Verification items for the finished model (mm, model axes). A direction names the side the tool comes from. Round coordinates to 2 decimals unless told otherwise and drop trailing zeros. Write each loop counter-clockwise with the first axis right and the second up, starting at its lowest first coordinate (ties: lowest second). Pieces come first, ordered by that corner, then holes.
from build123d import *

# Parameters (mm, degrees)
F0_W     = 9.545457
F0_H     = 70.051323
F1_DEPTH = 10
F3_DEPTH = 50
F0_W_2   = 6.466273
F4_DEPTH = 20
F6_DEPTH = 50


with BuildPart() as f1:
    # F0 (on Top) → F1 (new body)
    with BuildSketch(Plane.XY):
        with Locations((-40.414223, 12.239737)):
            Rectangle(F0_W, F0_H)
    extrude(amount=F1_DEPTH)

    # F2 (on Right) → F3 (cut)
    with BuildSketch(Plane.YZ):
        with BuildLine():
            ThreePointArc((-10.673997, 12.938293), (14.378322, 4.831678), (39.214806, 13.577245))
            Line((39.214806, 13.577245), (-10.673997, 12.938293))
        make_face()
    extrude(amount=-F3_DEPTH, mode=Mode.SUBTRACT)

    # F0 (on Top) → F4 (join)
    with BuildSketch(Plane.XY):
        with Locations((-32.408358, 12.239737)):
            Rectangle(F0_W_2, F0_H)
    extrude(amount=F4_DEPTH)

    # F5 (on Right) → F6 (cut)
    with BuildSketch(Plane.YZ):
        with BuildLine():
            Line((46.000224, 26.69229), (-19.578034, 26.722144))
            ThreePointArc((-19.578034, 26.722144), (13.203243, 9.459906), (46.000224, 26.69229))
        make_face()
    extrude(amount=-F6_DEPTH, mode=Mode.SUBTRACT)


solid = f1.part
Q1. Material ranges on line 1 along X through (y, z) = (33, 13.75); line 2 along Y through (x, z) = (-33.5, 18.5); line 3 along Z through (x, y) = (-40.25, 13), recorded low to high.
Recorded:
line 1: x = -35.64 to -29.18
line 2: y = -22.79 to -12.03, 38.47 to 47.27
line 3: z = 0 to 4.84
Q2. Sectioned sample at A-A (z = 13). Enter the section's corners in (x, y).
Recorded:
outline: (-35.64, -22.79) - (-29.18, -22.79) - (-29.18, -3.19) - (-35.64, -3.19) - close; (-35.64, 29.63) - (-29.18, 29.63) - (-29.18, 47.27) - (-35.64, 47.27) - close
Q3. Depth check by flat-ended pin: P1, Ø5, axis at y = 14.5, z = 10, coming from the +X side; P2, Ø3, axis at x = -35.5, y = 9.5, coming from the +Z side; P3, Ø6, axis at x = -40, y = 39.5, coming from the +Z side; P4, Ø5, axis at x = -43, z = 14, coming from the -Y side. Enter the tip coordinate at first touch or a pass-through.
Recorded:
P1: stops at x = -29.18
P2: stops at z = 9.8
P3: stops at z = 10
P4: passes through
Q4. Release check for a two-part mould opening along Y. For faces 4 (the flat face through (-40, -14, 10)), 5 (the flat face through (-36, 47.265, 8)), 6 (the flat face through (-35.641, 12, 9)) record: released by +Y, released by -Y, zero draft, split by the parting line, or undercut.
Recorded:
face 4: zero draft
face 5: released by +Y
face 6: undercut
Q5. Sectioned sample at B-B (x = -37.5). Enter the section's corners in (y, z).
Recorded:
outline: (-22.79, 0) - (47.27, 0) - (47.27, 10) - (33.82, 10) arc R41.14 cw to (-6.12, 10) - (-22.79, 10) - close
Q6. Tool access check on faces 1 (the flat face through (-32, 44, 20)), 2 (the flat face through (-40, 41, 10)), 3 (the cylindrical face through (-40.35, 13.56, 4.83)). Record the directions out of +Z, -Z, +X, -X, +Y, -Y that give a thin tool (end or side, any length) a straight path to the whole face; none if there is none.
Recorded:
face 1: +Z, +X, -X, +Y, -Y
face 2: +Z, -X, +Y, -Y
face 3: +Z, -X
Q7. Sectioned sample at C-C (y = -10). Enter the section's corners in (x, z).
Recorded:
outline: (-45.19, 0) - (-29.18, 0) - (-29.18, 16.94) - (-35.64, 16.94) - (-35.64, 10) - (-45.19, 10) - close
